Geometry check sheet. Reference: the model listing, model coordinates, mm. A direction names the side the tool comes from. Round coordinates to 2 decimals unless told otherwise and drop trailing zeros. Loops run counter-clockwise (first coordinate to the right, second up) from the corner with the lowest first, then second, coordinate; pieces in that order, holes last.
```python
from build123d import *

# Parameters (mm, degrees)
CROQUIS1_W              = 140
CROQUIS1_H              = 161
CROQUIS1_W_2            = 80
CROQUIS1_H_2            = 101
SALIENTE_EXTRUIR1_DEPTH = 2.5
CROQUIS2_W              = 85
CROQUIS2_H              = 106
CROQUIS2_W_2            = 80
CROQUIS2_H_2            = 101
SALIENTE_EXTRUIR2_DEPTH = 60
CROQUIS3_R              = 67.935631299
SALIENTE_EXTRUIR3_DEPTH = 500


with BuildPart() as part:
    # Croquis1 → Saliente-Extruir1 (new body)
    with BuildSketch(Plane.XY):
        with Locations((70, -80.5)):
            Rectangle(CROQUIS1_W, CROQUIS1_H)
        with Locations((70, -80.5)):
            Rectangle(CROQUIS1_W_2, CROQUIS1_H_2, mode=Mode.SUBTRACT)
    extrude(amount=SALIENTE_EXTRUIR1_DEPTH)

    # Croquis2 → Saliente-Extruir2 (add)
    with BuildSketch(Plane.XY.offset(2.5)):
        with Locations((70, -80.5)):
            Rectangle(CROQUIS2_W, CROQUIS2_H)
        with Locations((70, -80.5)):
            Rectangle(CROQUIS2_W_2, CROQUIS2_H_2, mode=Mode.SUBTRACT)
    extrude(amount=SALIENTE_EXTRUIR2_DEPTH)

    # Croquis3 → Saliente-Extruir3 (add)
    with BuildSketch(Plane.XY.offset(62.5)):
        with Locations(Location((70, -80.5, 0), (0, 0, 128.725665443))):
            Circle(CROQUIS3_R)
    extrude(amount=SALIENTE_EXTRUIR3_DEPTH)


solid = part.part
```
1) Sectioned sample at B-B, the plane x = 70. Record the cut outline in (y, z).
Report:
outline: (-161, 0) - (-131, 0) - (-131, 62.5) - (-30, 62.5) - (-30, 0) - (0, 0) - (0, 2.5) - (-27.5, 2.5) - (-27.5, 62.5) - (-12.56, 62.5) - (-12.56, 562.5) - (-148.44, 562.5) - (-148.44, 62.5) - (-133.5, 62.5) - (-133.5, 2.5) - (-161, 2.5) - close
2) Sectioned sample at C-C, the plane z = 138. Record the cut outline in (x, y).
Report:
outline: circle Ø135.87 at (70, -80.5)
3) Sectioned sample at A-A, the plane y = -80.5. Record the cut outline in (x, z).
Report:
outline: (0, 0) - (30, 0) - (30, 62.5) - (110, 62.5) - (110, 0) - (140, 0) - (140, 2.5) - (112.5, 2.5) - (112.5, 62.5) - (137.94, 62.5) - (137.94, 562.5) - (2.06, 562.5) - (2.06, 62.5) - (27.5, 62.5) - (27.5, 2.5) - (0, 2.5) - close
4) Sectioned sample at D-D, the plane x = 11.5. Record the cut outline in (y, z), then the cut area to 3 significant figures.
Report:
outline: (-161, 0) - (0, 0) - (0, 2.5) - (-161, 2.5) - close; (-115.04, 62.5) - (-45.96, 62.5) - (-45.96, 562.5) - (-115.04, 562.5) - close
area: 34,900 mm2
5) Scan lines: line 1 along Z through (x, y) = (56.5, -20.5); line 2 along Z through (x, y) = (49, -33.5); line 3 along Z through (x, y) = (131, -22). Record each from-to range of solid material in increasing order.
Report:
line 1: z = 0 to 2.5, 62.5 to 562.5
line 2: z = 62.5 to 562.5
line 3: z = 0 to 2.5
6) Access from +Z, -Z, +X, -X, +Y, -Y to the whole of each face (thin tool, end or side, straight path). Record for faces 1 (the face through (69, -133.5, 32)), 2 (the face through (125, -83, 62.5)), 3 (the face through (15, -79, 62.5)), 4 (the face through (70, -20, 62.5)), 5 (the face through (30, -81, 31)).
Report:
face 1: +X, -X, -Y
face 2: +X, +Y, -Y
face 3: -X, +Y, -Y
face 4: +X, -X, +Y
face 5: -Z
7) Mould release check, pull along X, two halves, no side actions. Record for faces 6 (the face through (65.504, -148.287, 309)), 7 (the face through (22, -79, 2.5)), 8 (the face through (70, -82, 62.5)): +X half, -X half, draft (parallel to the pull), parting line (faces both ways), or undercut.
Report:
face 6: parting line
face 7: draft
face 8: undercut
8) Gauge pin test, flat ends, axial feed: pin 1 (19 mm diameter, centred on x = 55, z = 38.5, fed in from -Y); pin 2 (10 mm diameter, centred on x = 18.5, z = 199, fed in from -Y); pin 3 (10 mm diameter, centred on y = -22.5, z = 210.5, fed in from +X). Record the tip position at first contact, or that the pin passes through.
Report:
pin 1: stops at y = -133.5
pin 2: stops at y = -130.03
pin 3: stops at x = 112.5
